Answer from the drawing. Dimensions are ordinates in mm from the lowest x, y and z of the part. A direction names the side the tool comes from. Coordinates: 2 decimals unless noted, no trailing zeros. Order: outer loops, then holes, each group sorted by start corner. A loop starts at its lowest first (then second) coordinate and runs counter-clockwise, first axis right, second up.
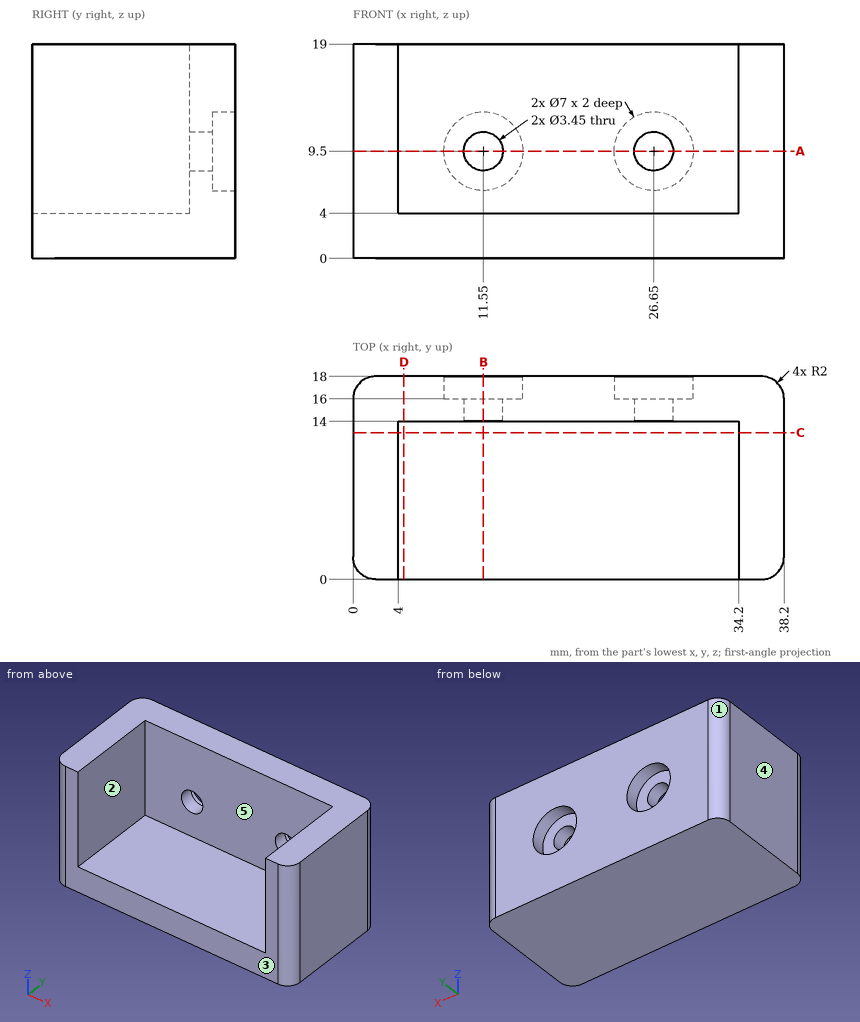
1) Section A-A (z = 9.5) is taken. Give the vertices of the cut face in (x, y) (3 decimals), then the cut area to 3 significant figures.
2) Each of these flat-tipped pins is pushed along its axis until it touches: P1, Ø3, axis at x = 26.65, z = 9.5, coming from the +Y side; P2, Ø5.5, axis at x = 27, z = 9.5, coming from the +Y side; P3, Ø4, axis at x = 11, z = 10.5, coming from the -Y side. Where does it stop, or does it pass through?
3) Consider L1, parallel to Z at x = 26.65, y = 15.4 (3 decimals); L2, parallel to Z at x = 26.65, y = 16.55; L3, parallel to X at y = 4.5, z = 14.5. Determine where each line is inside the solid, lowest interval first.
4) Determine the mould class of the marked faces 1, 2 and 3 for opening direction X: released by +X, released by -X, zero draft, split by the parting line, or undercut.
5) Section D-D (x = 4.5) is taken. Give the vertices of the cut face in (y, z).
6) Section B-B (x = 11.55) is taken. Give the vertices of the cut face in (y, z) (3 decimals).
7) A tool of negligible diameter and unlimited length cuts with its end or side. For the marked faces 4 and 5, from which of +Z, -Z, +X, -X, +Y, -Y can it reach the whole face along a straight path? Write none if from no direction.
8) Section C-C (y = 13) is taken. Give the vertices of the cut face in (x, z).
Filled sheet:
1. outline: (0, 2) arc R2 ccw to (2, 0) - (4, 0) - (4, 14) - (9.825, 14) - (9.825, 16) - (8.05, 16) - (8.05, 18) - (2, 18) arc R2 ccw to (0, 16) - close; (13.275, 14) - (24.925, 14) - (24.925, 16) - (23.15, 16) - (23.15, 18) - (15.05, 18) - (15.05, 16) - (13.275, 16) - close; (28.375, 14) - (34.2, 14) - (34.2, 0) - (36.2, 0) arc R2 ccw to (38.2, 2) - (38.2, 16) arc R2 ccw to (36.2, 18) - (30.15, 18) - (30.15, 16) - (28.375, 16) - close
1. area: 220 mm2
2. P1: passes through
2. P2: stops at y = 16
2. P3: stops at y = 14
3. L1: z = 0 to 7.775, 11.225 to 19
3. L2: z = 0 to 6, 13 to 19
3. L3: x = 0 to 4, 34.2 to 38.2
4. face 1: released by -X
4. face 2: undercut
4. face 3: zero draft
5. outline: (0, 0) - (18, 0) - (18, 19) - (14, 19) - (14, 4) - (0, 4) - close
6. outline: (0, 0) - (18, 0) - (18, 6) - (16, 6) - (16, 7.775) - (14, 7.775) - (14, 4) - (0, 4) - close; (14, 11.225) - (16, 11.225) - (16, 13) - (18, 13) - (18, 19) - (14, 19) - close
7. face 4: +Z, -Z, -X, +Y, -Y
7. face 5: +Z, -Y
8. outline: (0, 0) - (38.2, 0) - (38.2, 19) - (34.2, 19) - (34.2, 4) - (4, 4) - (4, 19) - (0, 19) - close
